Model file for the job. Use its own axes, mm. Give positions to 0.01 mm unless a question says otherwise; leave off trailing zeros. Order: outer loops, then holes, each group sorted by start corner. A loop starts at its lowest first (then second) coordinate and runs counter-clockwise, first axis right, second up. Notation, with made-up numbers: M -39,46 L -7,46 A33 ccw -7,75 Z; hole C 56.25,51 d2. An arc over 180 degrees is marked long. Return JSON: item names as keys, results as strings. Group by question number.
1. Slice it at C-C on z = -9. List the corners of the cut face in (x, y), then the cut area to 3 significant figures.
2. Slice it at D-D on x = -45. List the corners of the cut face in (y, z).
3. Pin check, flat tip, straight feed: pin 1 (1.5 mm diameter, centred on y = -2, z = -77, fed in from +X). Stop position of the tip, or through.
4. Wall check: probe 1 along X at (y, z) = (-1, -18); probe 2 along X at (y, z) = (-0.85, -63); probe 3 along X at (y, z) = (-1.2, -2). Give the ranges that are in metal, low to high. Write a range as [from, to].
5. Slice it at B-B on z = -51. List the corners of the cut face in (x, y), then the cut area to 3 significant figures.
6. Slice it at A-A on y = -2.5. List the corners of the cut face in (x, z) (1 decimal).
from build123d import *

# Parameters (mm, degrees)
F1_W     = 6
F1_H     = 3
F2_DEPTH = 3


with BuildPart() as f2:
    # F1 (on Front) → F2 (new body)
    with BuildSketch(Plane.XZ):
        Polygon((-49, 75), (49, 75), (0, 124), align=None)
        with BuildLine():
            Line((43, -75), (49, -75))
            Line((49, -75), (49, 0))
            ThreePointArc((49, 0), (47, 37.5), (49, 75))
            Line((49, 75), (-49, 75))
            ThreePointArc((-49, 75), (-47, 37.5), (-49, 0))
            Line((-49, 0), (-49, -75))
            Line((-49, -75), (-43, -75))
            Line((-43, -75), (-43, 0))
            Line((-43, 0), (-40, 0))
            Line((-40, 0), (-40, -35))
            ThreePointArc((-40, -35), (0, -28), (40, -35))
            Line((40, -35), (40, 0))
            Line((40, 0), (43, 0))
            Line((43, 0), (43, -75))
        make_face()
        with Locations((-46, -76.5)):
            Rectangle(F1_W, F1_H)
        with Locations((46, -76.5)):
            Rectangle(F1_W, F1_H)
        with BuildLine():
            Line((-49, -75), (-49, 0))
            ThreePointArc((-49, 0), (-51, -37.5), (-49, -75))
        make_face()
        with BuildLine():
            Line((49, 0), (49, -75))
            ThreePointArc((49, -75), (51, -37.5), (49, 0))
        make_face()
    extrude(amount=F2_DEPTH)


solid = f2.part
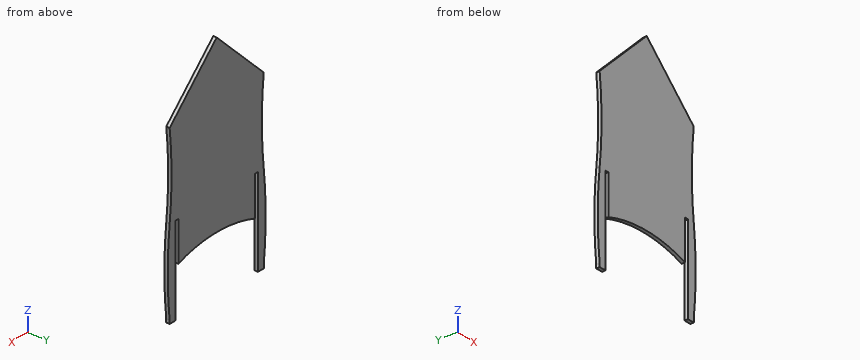
Result:
{
 "1": {"outline": "M -49.85,-3 L -43,-3 L -43,0 L -49.85,0 Z; M -40,-3 L 40,-3 L 40,0 L -40,0 Z; M 43,-3 L 49.85,-3 L 49.85,0 L 43,0 Z", "area": "281 mm2"},
 "2": {"outline": "M -3,-78 L 0,-78 L 0,79 L -3,79 Z"},
 "3": {"pin 1": "stops at x = 49"},
 "4": {"probe 1": "x = [-50.46, -43], [-40, 40], [43, 50.46]", "probe 2": "x = [-50.08, -43], [43, 50.08]", "probe 3": "x = [-49.21, -43], [-40, 40], [43, 49.21]"},
 "5": {"outline": "M -50.74,-3 L -43,-3 L -43,0 L -50.74,0 Z; M 43,-3 L 50.74,-3 L 50.74,0 L 43,0 Z", "area": "46.4 mm2"},
 "6": {"outline": "M -49,-78 L -43,-78 L -43,0 L -40,0 L -40,-35 A117.8 cw 40,-35 L 40,0 L 43,0 L 43,-78 L 49,-78 L 49,-75 A352.6 ccw 49,0 A352.6 cw 49,75 L 0,124 L -49,75 A352.6 cw -49,0 A352.6 ccw -49,-75 Z"}
}
